The listing builds one solid part. Answer for the finished solid, in the listing's coordinates (mm). A direction names the side the tool comes from. Coordinates: 2 decimals unless noted, no trailing zeros. Write each loop counter-clockwise with the first axis right and the second up, starting at its lowest first coordinate (ties: lowest second). Pieces come first, ordered by that corner, then holes.
```python
from build123d import *

# Parameters (mm, degrees)
PAD007_DEPTH         = 1
MIRRORED007_FACE34_W = 3
MIRRORED007_FACE34_H = 1
PAD008_DEPTH         = 20


with BuildPart() as part:
    # Sketch008 → Pad007 (new body)
    with BuildSketch(Plane.XY):
        with BuildLine():
            Line((0, 0.2), (0.6, 0.2))
            Line((0.6, 0.2), (0.6, 5))
            Line((1.496626, 4.505237), (0.6, 5))
            ThreePointArc((1.5, 4.156922), (1.599991, 4.332064), (1.496626, 4.505237))
            ThreePointArc((1.5, 4.156922), (1.4, 3.983717), (1.5, 3.810512))
            ThreePointArc((1.5, 3.464102), (1.6, 3.637307), (1.5, 3.810512))
            ThreePointArc((1.5, 3.464102), (1.4, 3.290897), (1.5, 3.117691))
            ThreePointArc((1.5, 2.771281), (1.6, 2.944486), (1.5, 3.117691))
            ThreePointArc((1.5, 2.771281), (1.4, 2.598076), (1.5, 2.424871))
            ThreePointArc((1.5, 2.078461), (1.6, 2.251666), (1.5, 2.424871))
            ThreePointArc((1.5, 2.078461), (1.4, 1.905256), (1.5, 1.732051))
            ThreePointArc((1.5, 1.385641), (1.6, 1.558846), (1.5, 1.732051))
            ThreePointArc((1.5, 1.385641), (1.4, 1.212436), (1.5, 1.03923))
            ThreePointArc((1.5, 0.69282), (1.6, 0.866025), (1.5, 1.03923))
            ThreePointArc((1.5, 0.69282), (1.4, 0.519615), (1.5, 0.34641))
            ThreePointArc((1.5, 0), (1.6, 0.173205), (1.5, 0.34641))
            Line((0, 0), (1.5, 0))
            Line((0, 0), (0, 0.2))
        make_face()
    pad007 = extrude(amount=PAD007_DEPTH)

    # Mirrored007: Pad007 across Sketch008 V_Axis
    add(pad007.mirror(Plane(origin=(0, 0, 0), x_dir=(0, 0, 1), z_dir=(1, 0, 0))))

    # Mirrored007 Face34 → Pad008 (add)
    with BuildSketch(Plane(origin=(0, 0, 0.5), x_dir=(-1, 0, 0), z_dir=(0, -1, 0))):
        Rectangle(MIRRORED007_FACE34_W, MIRRORED007_FACE34_H)
    extrude(amount=PAD008_DEPTH)


solid = part.part
```
(1) Section C-C, the plane y = -7.5 is taken. Write down the section's boundary in (x, z).
(2) Find the intervals of material crossed by probe 1 along Y at (x, z) = (-0.25, 0.55); probe 2 along X at (y, z) = (-12.75, 0.4); probe 3 along X at (y, z) = (2.75, 0.55), in increasing order.
(3) Which of the six approach directions +Z, -Z, +X, -X, +Y, -Y give full straight-line access (tool end or side, diameter ignored) to faces 5 (the flat face through (0.6, 2.6, 0.5)), 6 (the flat face through (0, -7, 0)), 7 (the flat face through (1.5, -9.9, 0.5))?
(4) For a pull along X with two mould halves and no side action, classify faces 1 (the flat face through (0, 0.2, 0.5)), 2 (the flat face through (-1.5, -9.9, 0.5)), 3 (the flat face through (0, -7, 1)), 4 (the flat face through (-0.6, 2.6, 0.5)) as pulls with the +X half, pulls with the -X half, needs draft (parallel to the pull), parting line crosses it, or undercut.
(5) Section B-B, the plane x = -0.3 is taken. Write down the section's boundary in (y, z).
(6) Each of these flat-tipped pins is pushed along its axis until it touches: pin 1 (0.5 mm diameter, centred on x = 0, z = 0.5, fed in from +Y); pin 2 (0.5 mm diameter, centred on y = -8, z = 0.5, fed in from +X). Where does it stop, or does it pass through?
Solution:
1. outline: (-1.5, 0) - (1.5, 0) - (1.5, 1) - (-1.5, 1) - close
2. probe 1: y = -20 to 0.2
2. probe 2: x = -1.5 to 1.5
2. probe 3: x = -1.47 to -0.6, 0.6 to 1.47
3. face 5: +Z, -Z, +Y
3. face 6: -Z, +X, -X, +Y, -Y
3. face 7: +Z, -Z, +X, -Y
4. face 1: undercut
4. face 2: pulls with the -X half
4. face 3: needs draft
4. face 4: undercut
5. outline: (-20, 0) - (0.2, 0) - (0.2, 1) - (-20, 1) - close
6. pin 1: stops at y = 0.2
6. pin 2: stops at x = 1.5
